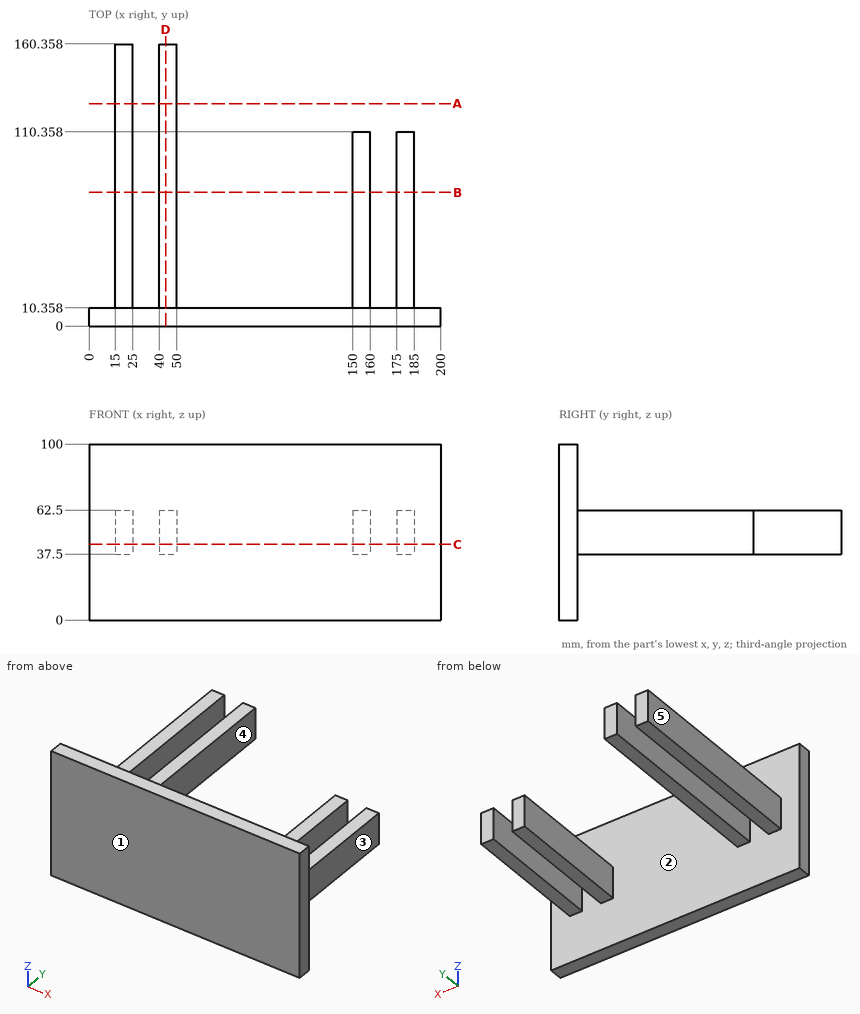
Job drawing, mm, ordinate dimensions from the low corner. One solid piece. A direction names the side the tool comes from. Give positions to 0.01 mm unless a question says otherwise; leave off trailing zeros. Loops run counter-clockwise (first coordinate to the right, second up) from the corner with the lowest first, then second, coordinate; pieces in that order, holes last. Notation, with made-up numbers: M 5.25,18.25 L 64.25,18.25 A18 ccw 64.25,53.25 Z; hole C 57.25,-15.75 d1. An arc over 180 degrees is marked long. Put each result on its own line as item: value. Start each with the question number.
1) 3-axis set-ups, long thin cutter, end or side, ignore diameter. For the marked faces 4 and 5: which of +Z, -Z, +X, -X, +Y, -Y reach the whole face in a straight line?
2) Saw through at A-A (y = 126.5). List the corners of the cut face in (x, z), then the cut area to 3 significant figures.
3) Saw through at D-D (x = 43.5). List the corners of the cut face in (y, z).
4) Pull direction X, two halves, no side cores. Call the marked faces 1, 2 and 3: +X half, -X half, draft (parallel to the pull), parting line (faces both ways), or undercut.
5) Flat gauge pins, fed straight in: pin 1 (20 mm diameter, centred on y = 60.5, z = 49.5, fed in from -X); pin 2 (6 mm diameter, centred on x = 160, z = 85.5, fed in from +Y); pin 3 (11 mm diameter, centred on x = 44, y = 65.5, fed in from -Z). Where does each tip first touch, or does it go through?
6) Saw through at C-C (z = 43). List the corners of the cut face in (x, y), then the cut area to 3 significant figures.
7) Probe probe 1 along X at (y, z) = (32, 62); probe 2 along Y at (x, z) = (135, 37.5); probe 3 along Y at (x, z) = (184, 38). List the from-to ranges inside material, lowest first.
8) Saw through at B-B (y = 76). List the corners of the cut face in (x, z), then the cut area to 3 significant figures.
Numbers:
1. face 4: +Z, -Z, +Y
1. face 5: +Z, -Z, -X, +Y
2. outline: M 15,37.5 L 25,37.5 L 25,62.5 L 15,62.5 Z; M 40,37.5 L 50,37.5 L 50,62.5 L 40,62.5 Z
2. area: 500 mm^2
3. outline: M 0,0 L 10.36,0 L 10.36,37.5 L 160.36,37.5 L 160.36,62.5 L 10.36,62.5 L 10.36,100 L 0,100 Z
4. face 1: draft
4. face 2: undercut
4. face 3: +X half
5. pin 1: x = 15
5. pin 2: y = 10.36
5. pin 3: z = 37.5
6. outline: M 0,0 L 200,0 L 200,10.36 L 185,10.36 L 185,110.36 L 175,110.36 L 175,10.36 L 160,10.36 L 160,110.36 L 150,110.36 L 150,10.36 L 50,10.36 L 50,160.36 L 40,160.36 L 40,10.36 L 25,10.36 L 25,160.36 L 15,160.36 L 15,10.36 L 0,10.36 Z
6. area: 7,070 mm^2
7. probe 1: 15 to 25, 40 to 50, 150 to 160, 175 to 185
7. probe 2: 0 to 10.36
7. probe 3: 0 to 110.36
8. outline: M 15,37.5 L 25,37.5 L 25,62.5 L 15,62.5 Z; M 40,37.5 L 50,37.5 L 50,62.5 L 40,62.5 Z; M 150,37.5 L 160,37.5 L 160,62.5 L 150,62.5 Z; M 175,37.5 L 185,37.5 L 185,62.5 L 175,62.5 Z
8. area: 1,000 mm^2
